from build123d import *

# Parameters (mm, degrees)
SKETCH_1_R           = 12.5
EXTRUDE_1_DEPTH      = 6
FILLET_1_R           = 3
FILLET_2_R           = 1
SKETCH_2_R           = 8
EXTRUDE_2_DEPTH      = 2.5
SKETCH_3_R           = 3.1
CUT_EXTRUDE_1_DEPTH  = 41.227129309
SKETCH_5_R           = 8
SKETCH_5_R_2         = 3.1
EXTRUDE_3_DEPTH      = 1.5
SKETCH_6_R           = 8
SKETCH_6_R_2         = 1.25
EXTRUDE_4_DEPTH      = 0.5
SKETCH_7_R           = 8
SKETCH_7_R_2         = 3.1
EXTRUDE_5_DEPTH      = 3.5
EXTRUDE_START        = -3.2
SKETCH_6_2_R         = 8
SKETCH_6_2_R_2       = 1.25
EXTRUDE_6_DEPTH      = 3.2
SKETCH_12_W          = 16
SKETCH_12_H          = 5
CUT_EXTRUDE_7_DEPTH  = 46.830983865
EXTRUDE_7_REACH      = 43.737
SKETCH_16_W          = 0.8
SKETCH_16_H          = 4
SKETCH_14_R          = 1.25
CUT_EXTRUDE_8_DEPTH  = 41.966107118
SKETCH_15_W          = 4.847698962
SKETCH_15_H          = 5
CUT_EXTRUDE_9_DEPTH  = 46.830983865
CUT_EXTRUDE_10_REACH = 42.697
SKETCH_17_R          = 1.55


with BuildPart() as part:
    # Sketch 1 → Extrude 1 (new body)
    with BuildSketch(Plane(origin=(0, 0, 0), x_dir=(1, 0, 0), z_dir=(0, 1, 0))):
        Circle(SKETCH_1_R)
        with BuildLine():
            Line((20.918584287, -9.767949192), (11.685855137, -4.437430532))
            ThreePointArc((11.685855137, -4.437430532), (10.825317547, -6.25), (9.685855137, -7.901532147))
            Line((9.685855137, -7.901532147), (18.918584287, -13.232050808))
            ThreePointArc((18.918584287, -13.232050808), (19.85043594, -14.446463525), (19.650635095, -15.964101615))
            Line((19.650635095, -15.964101615), (23.11473671, -17.964101615))
            ThreePointArc((23.11473671, -17.964101615), (23.714139245, -13.411187345), (20.918584287, -9.767949192))
        make_face()
        with BuildLine():
            Line((2, -23), (2, -12.338962679))
            ThreePointArc((2, -12.338962679), (0, -12.5), (-2, -12.338962679))
            Line((-2, -12.338962679), (-2, -23))
            ThreePointArc((-2, -23), (-2.585786438, -24.414213562), (-4, -25))
            Line((-4, -25), (-4, -29))
            ThreePointArc((-4, -29), (0.242640687, -27.242640687), (2, -23))
        make_face()
        with BuildLine():
            ThreePointArc((-9.685855137, -7.901532147), (-10.825317547, -6.25), (-11.685855137, -4.437430532))
            Line((-11.685855137, -4.437430532), (-20.918584287, -9.767949192))
            ThreePointArc((-20.918584287, -9.767949192), (-22.436222377, -9.967750037), (-23.650635095, -9.035898385))
            Line((-23.650635095, -9.035898385), (-27.11473671, -11.035898385))
            ThreePointArc((-27.11473671, -11.035898385), (-23.471498558, -13.831453343), (-18.918584287, -13.232050808))
            Line((-18.918584287, -13.232050808), (-9.685855137, -7.901532147))
        make_face()
        with BuildLine():
            Line((18.918584287, 13.232050808), (9.685855137, 7.901532147))
            ThreePointArc((9.685855137, 7.901532147), (10.825317547, 6.25), (11.685855137, 4.437430532))
            Line((11.685855137, 4.437430532), (20.918584287, 9.767949192))
            ThreePointArc((20.918584287, 9.767949192), (22.436222377, 9.967750037), (23.650635095, 9.035898385))
            Line((23.650635095, 9.035898385), (27.11473671, 11.035898385))
            ThreePointArc((27.11473671, 11.035898385), (23.471498558, 13.831453343), (18.918584287, 13.232050808))
        make_face()
        with BuildLine():
            Line((2, 12.338962679), (2, 23))
            ThreePointArc((2, 23), (2.585786438, 24.414213562), (4, 25))
            Line((4, 25), (4, 29))
            ThreePointArc((4, 29), (-0.242640687, 27.242640687), (-2, 23))
            Line((-2, 23), (-2, 12.338962679))
            ThreePointArc((-2, 12.338962679), (0, 12.5), (2, 12.338962679))
        make_face()
        with BuildLine():
            ThreePointArc((-11.685855137, 4.437430532), (-10.825317547, 6.25), (-9.685855137, 7.901532147))
            Line((-9.685855137, 7.901532147), (-18.918584287, 13.232050808))
            ThreePointArc((-18.918584287, 13.232050808), (-19.85043594, 14.446463525), (-19.650635095, 15.964101615))
            Line((-19.650635095, 15.964101615), (-23.11473671, 17.964101615))
            ThreePointArc((-23.11473671, 17.964101615), (-23.714139245, 13.411187345), (-20.918584287, 9.767949192))
            Line((-20.918584287, 9.767949192), (-11.685855137, 4.437430532))
        make_face()
    extrude(amount=EXTRUDE_1_DEPTH)

    # Fillet 1
    fillet_1_edges = [part.edges().sort_by_distance(p)[0] for p in [
        (-2, 3, 12.338962679),
        (-9.685855137, 3, 7.901532147),
        (-11.685855137, 3, 4.437430532),
        (-11.685855137, 3, -4.437430532),
        (-9.685855137, 3, -7.901532147),
        (-2, 3, -12.338962679),
        (2, 3, -12.338962679),
        (9.685855137, 3, -7.901532147),
        (11.685855137, 3, -4.437430532),
        (11.685855137, 3, 4.437430532),
        (9.685855137, 3, 7.901532147),
        (2, 3, 12.338962679),
    ]]
    fillet(fillet_1_edges, radius=FILLET_1_R)

    # Fillet 2
    fillet_2_edges = [part.edges().sort_by_distance(p)[0] for p in [
        (-4, 3, 29),
        (-4, 3, 25),
        (-27.11473671, 3, 11.035898385),
        (-23.650635095, 3, 9.035898385),
        (-23.11473671, 3, -17.964101615),
        (-19.650635095, 3, -15.964101615),
        (4, 3, -29),
        (4, 3, -25),
        (27.11473671, 3, -11.035898385),
        (23.650635095, 3, -9.035898385),
        (23.11473671, 3, 17.964101615),
        (19.650635095, 3, 15.964101615),
    ]]
    fillet(fillet_2_edges, radius=FILLET_2_R)

    # Sketch 2 → Extrude 2 (add)
    with BuildSketch(Plane(origin=(0, 0, 0), x_dir=(1, 0, 0), z_dir=(0, 1, 0))):
        with Locations(Location((0, 0, 0), (0, 0, 270))):
            Circle(SKETCH_2_R)
    extrude(amount=-EXTRUDE_2_DEPTH)

    # Sketch 3 → Cut-Extrude 1 (cut, through all)
    with BuildSketch(Plane(origin=(0, -2.5, 0), x_dir=(-1, 0, 0), z_dir=(0, -1, 0))):
        with Locations(Location((0, 0, 0), (0, 0, 90))):
            Circle(SKETCH_3_R)
    extrude(amount=-CUT_EXTRUDE_1_DEPTH, mode=Mode.SUBTRACT)

    # Sketch 5 → Extrude 3 (add)
    with BuildSketch(Plane(origin=(0, 6, 0), x_dir=(1, 0, 0), z_dir=(0, 1, 0))):
        with Locations(Location((0, 0, 0), (0, 0, 270))):
            Circle(SKETCH_5_R)
        with Locations(Location((0, 0, 0), (0, 0, 90))):
            Circle(SKETCH_5_R_2, mode=Mode.SUBTRACT)
    extrude(amount=EXTRUDE_3_DEPTH)

    # Sketch 6 → Extrude 4 (add)
    with BuildSketch(Plane(origin=(0, 7.5, 0), x_dir=(1, 0, 0), z_dir=(0, 1, 0))):
        with Locations(Location((0, 0, 0), (0, 0, 270))):
            Circle(SKETCH_6_R)
        with Locations(Location((0, 0, 0), (0, 0, 270))):
            Circle(SKETCH_6_R_2, mode=Mode.SUBTRACT)
    extrude(amount=EXTRUDE_4_DEPTH)

    # Sketch 7 → Extrude 5 (add)
    with BuildSketch(Plane(origin=(0, 8, 0), x_dir=(1, 0, 0), z_dir=(0, 1, 0))):
        with Locations(Location((0, 0, 0), (0, 0, 270))):
            Circle(SKETCH_7_R)
        with Locations(Location((0, 0, 0), (0, 0, 90))):
            Circle(SKETCH_7_R_2, mode=Mode.SUBTRACT)
    extrude(amount=EXTRUDE_5_DEPTH)

    # Sketch 6_2 → Extrude 6 (add)
    with BuildSketch(Plane(origin=(0, 7.5, 0), x_dir=(1, 0, 0), z_dir=(0, 1, 0)).offset(EXTRUDE_START)):
        with Locations(Location((0, 0, 0), (0, 0, 270))):
            Circle(SKETCH_6_2_R)
        with Locations(Location((0, 0, 0), (0, 0, 270))):
            Circle(SKETCH_6_2_R_2, mode=Mode.SUBTRACT)
    extrude(amount=EXTRUDE_6_DEPTH)

    # Sketch 12 → Cut-Extrude 7 (cut, through all)
    with BuildSketch(Plane(origin=(7, 0, 0), x_dir=(0, 0, -1), z_dir=(1, 0, 0))):
        with Locations((0, -2.5)):
            Rectangle(SKETCH_12_W, SKETCH_12_H)
    extrude(amount=CUT_EXTRUDE_7_DEPTH, mode=Mode.SUBTRACT)

    # Sketch 16 → Extrude 7 (add, up to next)
    with BuildSketch(Plane.XZ.offset(2.5), mode=Mode.PRIVATE) as extrude_7_sk1:
        with Locations((3.1, 0)):
            Rectangle(SKETCH_16_W, SKETCH_16_H)
    extrude_7_tool1 = extrude(extrude_7_sk1.sketch, amount=-EXTRUDE_7_REACH, mode=Mode.PRIVATE) - part.part
    add(extrude_7_tool1.solids().sort_by_distance((3.1, -2.5, 0))[0])

    # Sketch 14 → Cut-Extrude 8 (cut, through all)
    with BuildSketch(Plane(origin=(0, 0, 0), x_dir=(0, 0, -1), z_dir=(1, 0, 0))):
        with Locations(Location((0, 0, 0), (0, 0, 180))):
            Circle(SKETCH_14_R)
    extrude(amount=CUT_EXTRUDE_8_DEPTH, mode=Mode.SUBTRACT)

    # Sketch 15 → Cut-Extrude 9 (cut, through all)
    with BuildSketch(Plane(origin=(7, 0, 0), x_dir=(0, 0, -1), z_dir=(1, 0, 0))):
        Rectangle(SKETCH_15_W, SKETCH_15_H)
    extrude(amount=CUT_EXTRUDE_9_DEPTH, mode=Mode.SUBTRACT)

    # Sketch 17 → Cut-Extrude 10 (cut, up to next)
    with BuildSketch(Plane(origin=(0, 8, 0), x_dir=(1, 0, 0), z_dir=(0, 1, 0)), mode=Mode.PRIVATE) as cut_extrude_10_sk1:
        with Locations(Location((0, 0, 0), (0, 0, 270))):
            Circle(SKETCH_17_R)
    cut_extrude_10_tool1 = extrude(cut_extrude_10_sk1.sketch, amount=-CUT_EXTRUDE_10_REACH, mode=Mode.PRIVATE) & part.part
    add(cut_extrude_10_tool1.solids().sort_by_distance((0, 8, 0))[0], mode=Mode.SUBTRACT)


solid = part.part
Geometry: final body of the model. Coordinates: model frame, mm. A direction names the side the tool comes from. Coordinates: 2 decimals unless noted, no trailing zeros. Order: outer loops, then holes, each group sorted by start corner. A loop starts at its lowest first (then second) coordinate and runs counter-clockwise, first axis right, second up.
1) Set-up query: faces 1 (the cylindrical face through (-2.357, 2.958, 24.141)), 2 (the cylindrical face through (-3.1, 0.9, -0.1)), 3 (the cylindrical face through (6.22, 2.958, 10.842)), 4 (the cylindrical face through (-0.931, 9.726, -2.957)). Return all of +Z, -Z, +X, -X, +Y, -Y with unobstructed straight access to the full face (end or side cutting, diameter ignored); none if empty.
Result sheet:
face 1: -X, +Y, -Y
face 2: -Y
face 3: +Z, +Y, -Y
face 4: +Y
2) Section A-A (z = 0). Return loops of the section in (x, y), then the cut area to 3 significant figures.
Result sheet:
outline: (-12.5, 0) - (-8, 0) - (-8, -2.5) - (-3.1, -2.5) - (-3.1, 4.3) - (-1.55, 4.3) - (-1.55, 8) - (-3.1, 8) - (-3.1, 11.5) - (-8, 11.5) - (-8, 6) - (-12.5, 6) - close; (1.55, 4.3) - (2.7, 4.3) - (2.7, 1.25) - (7, 1.25) - (7, 2.5) - (12.5, 2.5) - (12.5, 6) - (8, 6) - (8, 11.5) - (3.1, 11.5) - (3.1, 8) - (1.55, 8) - close; (2.7, -2.5) - (7, -2.5) - (7, -1.25) - (2.7, -1.25) - close
area: 178 mm2
3) Draft query along Z for faces 5 (the flat face through (10, 1, -2.424)), 6 (the flat face through (-8, 6, -2)), 7 (the cylindrical face through (23.55, 2.96, 12.89)), 8 (the cylindrical face through (6.28, 2.96, -10.81)). Return one class per face: released by +Z, released by -Z, zero draft, split by the parting line, or undercut.
Result sheet:
face 5: undercut
face 6: zero draft
face 7: undercut
face 8: released by -Z
4) Section B-B (y = 10.75). Return loops of the section in (x, z).
Result sheet:
outline: circle Ø16 at (0, 0); hole circle Ø6.2 at (0, 0)
5) Section C-C (x = 0). Return loops of the section in (y, z).
Result sheet:
outline: (-2.5, -8) - (0, -8) - (0, -27.47) - (6, -27.47) - (6, -8) - (11.5, -8) - (11.5, -3.1) - (8, -3.1) - (8, -1.55) - (4.3, -1.55) - (4.3, -3.1) - (-2.5, -3.1) - close; (-2.5, 3.1) - (4.3, 3.1) - (4.3, 1.55) - (8, 1.55) - (8, 3.1) - (11.5, 3.1) - (11.5, 8) - (6, 8) - (6, 27.47) - (0, 27.47) - (0, 8) - (-2.5, 8) - close
6) First-contact query: P1, Ø6, axis at y = 1, z = 15, coming from the +X side; P2, Ø1.7, axis at y = 2, z = -27, coming from the +X side; P3, Ø1.5, axis at y = 0, z = 0, coming from the +X side. Flat tips, straight axial feed; report the tip coordinate or a pass-through.
Result sheet:
P1: stops at x = 23.92
P2: stops at x = 4
P3: stops at x = -3.01
7) Section D-D (x = 9). Return loops of the section in (y, z), then the cut area to 3 significant figures.
Result sheet:
outline: (0, -8.92) - (6, -8.92) - (6, 8.92) - (0, 8.92) - (0, 2.42) - (2.5, 2.42) - (2.5, -2.42) - (0, -2.42) - close
area: 94.9 mm2
8) Ray query, probe 1 along X at (y, z) = (9.2, 0); probe 2 along X at (y, z) = (5.75, 11); probe 3 along Y at (x, z) = (4.45, 0). Return the intervals inside material, ascending.
Result sheet:
probe 1: x = -8 to -3.1, 3.1 to 8
probe 2: x = -26.6 to -15.05, -5.94 to 5.94, 15.05 to 22.42
probe 3: y = -2.5 to -1.25, 1.25 to 11.5
